Can you work these out from the model? Positions are in its coordinate system, mm. A direction names the side the tool comes from. Give positions to 0.01 mm unless a question says otherwise; leave off trailing zeros. Order: outer loops, then holes, each group sorted by start corner. A loop starts at its lowest first (then second) coordinate and runs counter-clockwise, first axis right, second up. Notation, with made-up numbers: (-32, 50) - (5, 50) arc R23 ccw to (5, 73) - close; hole circle Ø1 at (46, 48.5). An arc over 180 degrees is marked (long way). Use one line per item in the form item = value. Start each with the question number.
1) For pin 1 (4.5 mm diameter, centred on x = 10, y = 0, fed in from +Z); pin 2 (6.5 mm diameter, centred on x = -10, y = 0, fed in from -Z), each with a flat end and sliding along its axis, tell me the tip position at first contact or that it passes through.
2) Suppose I cut it at D-D, the plane z = 2. State how many separate pieces and enclosed holes the cut face has, and give its area (3 significant figures).
3) We'd pull the mould along X, two halves only. Please class faces 4 (the cylindrical face through (-16.072, -28.167, 3.131)), 5 (the flat face through (25, -27, 3)), 6 (the flat face through (0, -25, 6.35)), 7 (the cylindrical face through (-2.027, -8.141, 4.797)): released by +X, released by -X, zero draft, split by the parting line, or undercut.
4) Please list where these lines run through material, in increasing order: probe 1 along X at (y, z) = (-50.5, 0.75); probe 2 along Y at (x, z) = (0, 3.9); probe 3 along Y at (x, z) = (0, 1.95).
5) Suppose I cut it at C-C, the plane x = 10. Write out the boundary of the cut face in (y, z).
6) Suppose I cut it at B-B, the plane y = -43. Write out the boundary of the cut face in (x, z), and give its area (3 significant figures).
7) Which directions (+Z, -Z, +X, -X, +Y, -Y) give clear straight access to the entire face, cutting with the end or side of a thin tool? Please do faces 1 (the cylindrical face through (-14.77, 1.5, 1.58)), 2 (the cylindrical face through (-15.932, -73.164, 3.131)), 3 (the flat face through (0, -76.987, 3)).
8) Suppose I cut it at A-A, the plane x = 0. Write out the boundary of the cut face in (y, z).
```python
from build123d import *

# Parameters (mm, degrees)
BOSS_EXTRUDE1_DEPTH                            = 6.35
CSK_FOR_6_FLAT_HEAD_MACHINE_SCREW2_D           = 4.3053
CSK_FOR_6_FLAT_HEAD_MACHINE_SCREW2_CSINK_D     = 9.7361756
CSK_FOR_6_FLAT_HEAD_MACHINE_SCREW2_CSINK_ANGLE = 82
CBORE_FOR_M5_SHCS1_D                           = 5.5
CBORE_FOR_M5_SHCS1_CBORE_D                     = 10
CBORE_FOR_M5_SHCS1_CBORE_DEPTH                 = 3.2


with BuildPart() as part:
    # Sketch1 → Boss-Extrude1 (new body)
    with BuildSketch(Plane.XY):
        Polygon((25, -76.9874), (25, 25), (-25, 25), (-25, -76.9874), (0, -76.9874), align=None)
        with BuildLine():
            ThreePointArc((-19.177, -31.341450548), (-16.002, -28.166450548), (-12.827, -31.341450548))
            Line((-12.827, -31.341450548), (-12.827, -69.9897))
            ThreePointArc((-12.827, -69.9897), (-16.002, -73.1647), (-19.177, -69.9897))
            Line((-19.177, -69.9897), (-19.177, -31.341450548))
        make_face(mode=Mode.SUBTRACT)
        with BuildLine():
            ThreePointArc((12.827, -31.341450548), (16.002, -28.166450548), (19.177, -31.341450548))
            Line((19.177, -31.341450548), (19.177, -69.9897))
            ThreePointArc((19.177, -69.9897), (16.002, -73.1647), (12.827, -69.9897))
            Line((12.827, -69.9897), (12.827, -31.341450548))
        make_face(mode=Mode.SUBTRACT)
    extrude(amount=BOSS_EXTRUDE1_DEPTH)

    # CSK for #6 Flat Head Machine Screw2 (through all)
    with Locations(Plane.XY.offset(6.35)):
        with Locations((18.904, 5.04825), (18.904, -5.04825)):
            CounterSinkHole(CSK_FOR_6_FLAT_HEAD_MACHINE_SCREW2_D / 2, CSK_FOR_6_FLAT_HEAD_MACHINE_SCREW2_CSINK_D / 2, counter_sink_angle=CSK_FOR_6_FLAT_HEAD_MACHINE_SCREW2_CSINK_ANGLE)

    # CBORE for M5 SHCS1 (through all)
    with Locations(Plane(origin=(0, 0, 0), x_dir=(-1, 0, 0), z_dir=(0, 0, -1))):
        with Locations((0, 10), (-10, 0), (0, -10), (10, 0)):
            CounterBoreHole(CBORE_FOR_M5_SHCS1_D / 2, CBORE_FOR_M5_SHCS1_CBORE_D / 2, CBORE_FOR_M5_SHCS1_CBORE_DEPTH)


solid = part.part
```
Result sheet:
q1.pin_1 = through
q1.pin_2 = 3.2
q2.separate_pieces = 1
q2.enclosed_holes = 8
q2.area = 4,200 mm²
q3.face_4 = undercut
q3.face_5 = released by +X
q3.face_6 = zero draft
q3.face_7 = undercut
q4.probe_1 = -25 to -19.18, -12.83 to 12.83, 19.18 to 25
q4.probe_2 = -76.99 to -12.75, -7.25 to 7.25, 12.75 to 25
q4.probe_3 = -76.99 to -15, -5 to 5, 15 to 25
q5.outline = (-76.99, 0) - (-5, 0) - (-5, 3.2) - (-2.75, 3.2) - (-2.75, 6.35) - (-76.99, 6.35) - close; (2.75, 3.2) - (5, 3.2) - (5, 0) - (25, 0) - (25, 6.35) - (2.75, 6.35) - close
q6.outline = (-25, 0) - (-19.18, 0) - (-19.18, 6.35) - (-25, 6.35) - close; (-12.83, 0) - (12.83, 0) - (12.83, 6.35) - (-12.83, 6.35) - close; (19.18, 0) - (25, 0) - (25, 6.35) - (19.18, 6.35) - close
q6.area = 237 mm²
q7.face_1 = -Z
q7.face_2 = +Z, -Z
q7.face_3 = +Z, -Z, +X, -X, -Y
q8.outline = (-76.99, 0) - (-15, 0) - (-15, 3.2) - (-12.75, 3.2) - (-12.75, 6.35) - (-76.99, 6.35) - close; (-7.25, 3.2) - (-5, 3.2) - (-5, 0) - (5, 0) - (5, 3.2) - (7.25, 3.2) - (7.25, 6.35) - (-7.25, 6.35) - close; (12.75, 3.2) - (15, 3.2) - (15, 0) - (25, 0) - (25, 6.35) - (12.75, 6.35) - close
